Print and shaded views of the part. All mm, measured from the part's lowest x, y and z. Round coordinates to 2 decimals unless told otherwise and drop trailing zeros. Loops run counter-clockwise (first coordinate to the right, second up) from the corner with the lowest first, then second, coordinate; pieces in that order, holes last. Notation, with made-up numbers: (38.25, 22) - (83.25, 22) arc R20 cw to (83.25, 38) - close; hole circle Ø5 at (-36, 79.5). An arc over 180 degrees is marked (long way). Put each result on its own line as item: value. Start each with the question number.
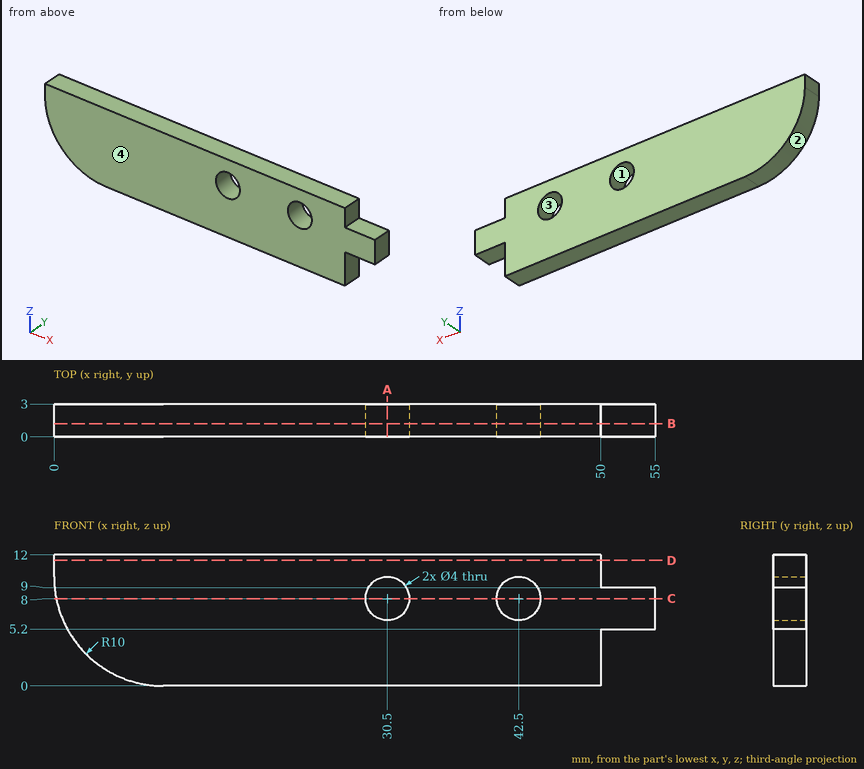
Item 1: Slice it at A-A (x = 30.5). Give the cut face in (y, z).
Item 2: Slice it at C-C (z = 8). Give the cut face in (x, y).
Item 3: Drill centre lines: probe 1 along X at (y, z) = (1.5, 6.5); probe 2 along X at (y, z) = (1.7, 7.75); probe 3 along Z at (x, y) = (42.5, 2.3). Where is each one in solid material? Low to high. Write a range as [from, to].
Item 4: Two-plate mould, pull along X, no slides. Class the marked faces 1, 2, 3 and 4: pulls with the +X half, pulls with the -X half, needs draft (parallel to the pull), parting line crosses it, or undercut.
Item 5: Slice it at D-D (z = 11.5). Give the cut face in (x, y), plus the area to 3 significant figures.
Item 6: Slice it at B-B (y = 1.2). Give the cut face in (x, z), plus the area to 3 significant figures.
Item 7: Drop flat-ended pins along their axis: pin 1 Ø1.5 at (x, y) = (53, 1.5) entering from +Z; pin 2 Ø0.9 at (y, z) = (1.5, 11) entering from +X. Give the stop position or say it passes through.
Computed values:
1. outline: (0, 0) - (3, 0) - (3, 6) - (0, 6) - close; (0, 10) - (3, 10) - (3, 12) - (0, 12) - close
2. outline: (0.2, 0) - (28.5, 0) - (28.5, 3) - (0.2, 3) - close; (32.5, 0) - (40.5, 0) - (40.5, 3) - (32.5, 3) - close; (44.5, 0) - (55, 0) - (55, 3) - (44.5, 3) - close
3. probe 1: x = [0.63, 29.18], [31.82, 41.18], [43.82, 55]
3. probe 2: x = [0.26, 28.52], [32.48, 40.52], [44.48, 55]
3. probe 3: z = [0, 6], [10, 12]
4. face 1: undercut
4. face 2: pulls with the -X half
4. face 3: undercut
4. face 4: needs draft
5. outline: (0, 0) - (50, 0) - (50, 3) - (0, 3) - close
5. area: 150 mm^2
6. outline: (0, 10) arc R10 ccw to (10, 0) - (50, 0) - (50, 5.2) - (55, 5.2) - (55, 9) - (50, 9) - (50, 12) - (0, 12) - close; hole circle Ø4 at (30.5, 8); hole circle Ø4 at (42.5, 8)
6. area: 572 mm^2
7. pin 1: stops at z = 9
7. pin 2: stops at x = 50
